from build123d import *

# Parameters (mm, degrees)
SKETCH046_R     = 2.5
PAD023_DEPTH    = 2.5
SKETCH047_R     = 5
PAD024_DEPTH    = 3
FILLET003_R     = 1.5
SKETCH049_R     = 2.5
PAD025_DEPTH    = 4
SKETCH050_R     = 1.5
POCKET026_DEPTH = 4
SKETCH088_W     = 1.5
SKETCH088_H     = 5
PAD052_DEPTH    = 0.2


with BuildPart() as part:
    # Sketch046 → Pad023 (new body)
    with BuildSketch(Plane(origin=(0, 0, 30), x_dir=(1, 0, 0), z_dir=(0, 0, -1))):
        with Locations((101, 55)):
            Circle(SKETCH046_R)
    extrude(amount=-PAD023_DEPTH)

    # Sketch047 (on Face3 of Pad023) → Pad024 (join)
    with BuildSketch(Plane.XY.offset(32.5)):
        with Locations((101, -55)):
            Circle(SKETCH047_R)
    extrude(amount=PAD024_DEPTH)

    # Fillet003
    fillet003_edges = [part.edges().sort_by_distance(p)[0] for p in [
        (96, -55, 35.5),
    ]]
    fillet(fillet003_edges, radius=FILLET003_R)

    # Sketch049 → Pad025 (join)
    with BuildSketch(Plane(origin=(0, 0, 30), x_dir=(1, 0, 0), z_dir=(0, 0, -1))):
        with Locations((101, 55)):
            Circle(SKETCH049_R)
    extrude(amount=PAD025_DEPTH)

    # Sketch050 (on Face17 of Pad025) → Pocket026 (cut)
    with BuildSketch(Plane(origin=(0, 0, 26), x_dir=(1, 0, 0), z_dir=(0, 0, -1))):
        with Locations((101, 55)):
            Circle(SKETCH050_R)
    extrude(amount=-POCKET026_DEPTH, mode=Mode.SUBTRACT)


with BuildPart() as part_1:
    # Body002 placement: moved
    add(part.part.moved(Location((75, 0, 0))))

    # Sketch088 (on Face4 of Clone001) → Pad052 (new body)
    with BuildSketch(Plane(origin=(75, 0, 35.5), x_dir=(1, 0, 0), z_dir=(0, 0, 1))):
        with Locations((99.75, -55)):
            Rectangle(SKETCH088_W, SKETCH088_H)
        with Locations((102.25, -55)):
            Rectangle(SKETCH088_W, SKETCH088_H)
    extrude(amount=PAD052_DEPTH)


with BuildPart() as part_2:
    # Body010 placement: moved
    add(part_1.part.moved(Location((-145.5, 0, 0))))


solid = part_2.part
Could you check a few things on this model? Use its own coordinates, in mm. A direction names the side the tool comes from. Give positions to 0.01 mm unless a question says otherwise; leave off trailing zeros. Order: outer loops, then holes, each group sorted by start corner. A loop starts at its lowest first (then second) coordinate and runs counter-clockwise, first axis right, second up.
Item 1: If we section it at D-D, the plane z = 30.5: Write out the boundary of the cut face in (x, y).
Item 2: If we section it at B-B, the plane y = -55: Write out the boundary of the cut face in (x, z), plus the area to 3 significant figures.
Item 3: If we mould it in two halves opening along Y, with no side actions, what happens to faces 3 (the face through (30, -55, 30)), 4 (the face through (30.5, -55, 35.5)), 5 (the face through (26.815, -51.621, 33.24))? For each: pulls with the +Y half, pulls with the -Y half, needs draft (parallel to the pull), parting line crosses it, or undercut.
Item 4: If we section it at C-C, the plane z = 28: Write out the boundary of the cut face in (x, y).
Item 5: For faces 1 (the face through (29.3, -54.1, 28)), 2 (the face through (32, -55, 35.7)), which set-ups out of +Z, -Z, +X, -X, +Y, -Y let a thin tool reach every point of the face, with its end or its side?
Item 6: If we section it at A-A, the plane x = 30.5: Write out the boundary of the cut face in (y, z), plus the area to 3 significant figures.
Item 7: I need wall thicknesses on line 1 (X direction, y = -55, z = 26.8); line 2 (Y direction, x = 30.5, z = 28.1); line 3 (Z direction, x = 31, y = -58.25). Which ranges of each line are inside material? Lowest first, please.
Item 8: I'm going to push flat-ended pins straight in: pin 1 (3 mm diameter, centred on y = -51, z = 33, fed in from +X); pin 2 (5 mm diameter, centred on x = 26.5, z = 33, fed in from +Y); pin 3 (1.5 mm diameter, centred on y = -52, z = 33.5, fed in from +X). Where does each tip first touch, or does it pass through?
Values:
1. outline: circle Ø5 at (30.5, -55)
2. outline: (25.5, 32.5) - (28, 32.5) - (28, 26) - (29, 26) - (29, 30) - (32, 30) - (32, 26) - (33, 26) - (33, 32.5) - (35.5, 32.5) - (35.5, 34) arc R1.5 ccw to (34, 35.5) - (32.5, 35.5) - (32.5, 35.7) - (31, 35.7) - (31, 35.5) - (30, 35.5) - (30, 35.7) - (28.5, 35.7) - (28.5, 35.5) - (27, 35.5) arc R1.5 ccw to (25.5, 34) - close
2. area: 50.1 mm2
3. face 3: undercut
3. face 4: needs draft
3. face 5: parting line crosses it
4. outline: circle Ø5 at (30.5, -55); hole circle Ø3 at (30.5, -55)
5. face 1: -Z
5. face 2: +Z, +X, -X, +Y, -Y
6. outline: (-60, 32.5) - (-57.5, 32.5) - (-57.5, 26) - (-56.5, 26) - (-56.5, 30) - (-53.5, 30) - (-53.5, 26) - (-52.5, 26) - (-52.5, 32.5) - (-50, 32.5) - (-50, 34) arc R1.5 ccw to (-51.5, 35.5) - (-58.5, 35.5) arc R1.5 ccw to (-60, 34) - close
6. area: 49.5 mm2
7. line 1: x = 28 to 29, 32 to 33
7. line 2: y = -57.5 to -56.5, -53.5 to -52.5
7. line 3: z = 32.5 to 35.5
8. pin 1: stops at x = 34.83
8. pin 2: stops at y = -50.23
8. pin 3: stops at x = 34.97
